Autodesk Inventor part; units mm, degrees
ref_plane "YZ Plane" through (0, 0, 0) normal (1, 0, 0) x (0, 1, 0)
ref_plane "XZ Plane" through (0, 0, 0) normal (0, 1, 0) x (-1, 0, 0)
ref_plane "XY Plane" through (0, 0, 0) normal (0, 0, 1) x (1, 0, 0)
sketch "Sketch1" plane through (0, 0, 0) normal (1, 0, 0) x (0, 1, 0)
  line L0 (0, 0) -> (50.8, 0) construction
  line L1 (50.8, 0) -> (50.8, -25.4) construction
  line L2 (50.8, -25.4) -> (0, -25.4) construction
  line L3 (0, -25.4) -> (0, 0) construction
  line L4 (12.7, -25.4) -> (139.7, -25.4) construction
  line L5 (139.7, -25.4) -> (139.7, -111.252) construction
  line L6 (139.7, -111.252) -> (12.7, -111.252) construction
  line L7 (12.7, -111.252) -> (12.7, -25.4) construction
  line L8 (80.9625, -111.252) -> (665.1625, -111.252) construction
  line L9 (665.1625, -111.252) -> (665.1625, -320.802) construction
  line L10 (665.1625, -320.802) -> (80.9625, -320.802) construction
  line L11 (80.9625, -320.802) -> (80.9625, -111.252) construction
  point P0 (0, -12.7)
  dimension "d0" = 50.8
  dimension "d1" = 25.4
  dimension "d2" = 12.7
  dimension "d3" = 85.852
  dimension "d4" = 127
  dimension "d5" = 80.9625
  dimension "d6" = 209.55
  dimension "d7" = 584.2
sketch "Sketch2" plane through (0, 0, 0) normal (1, 0, 0) x (0, 1, 0)
  line L0 (139.7, -25.4) -> (139.7, -111.252) construction
  line L1 (80.9625, -320.802) -> (80.9625, -111.252) construction
  line L2 (139.7, -111.252) -> (12.7, -111.252) construction
  line L3 (50.8, 0) -> (50.8, -25.4) construction
  line L4 (12.7, -25.4) -> (139.7, -25.4) construction
  line L5 (12.7, -111.252) -> (12.7, -25.4) construction
  line L6 (50.8, -25.4) -> (0, -25.4) construction
  line L7 (0, -25.4) -> (0, 0) construction
  line L8 (0, 0) -> (50.8, 0) construction
  line L9 (665.1625, -320.802) -> (80.9625, -320.802) construction
  line L10 (80.9625, -111.252) -> (665.1625, -111.252) construction
  line L11 (665.1625, -111.252) -> (665.1625, -320.802) construction
  line L12 (50.8, -25.4) -> (190.5, -25.4) construction
  line L13 (190.5, -25.4) -> (190.5, 0) construction
  line L14 (190.5, 0) -> (50.8, 0) construction
  line L15 (50.8, 0) -> (50.8, -25.4) construction
  line L16 (165.1, -12.7) -> (165.1, -216.027) construction
  line L17 (165.1, -216.027) -> (80.9625, -216.027) construction
  line L18 (80.9625, -225.552) -> (174.625, -225.552)
  line L19 (174.625, -225.552) -> (174.625, -12.7)
  line L20 (80.9625, -206.502) -> (155.575, -206.502)
  line L21 (155.575, -206.502) -> (155.575, -12.7)
  line L22 (80.9625, -206.502) -> (80.9625, -225.552)
  arc A0 (174.625, -12.7) -> (155.575, -12.7) centre (165.1, -12.7) ccw
  point P0 (0, -12.7)
  point P1 (190.5, -12.7)
  dimension "d8" = 50.8
  dimension "d9" = 25.4
  dimension "d10" = 9.525
  dimension "d11" = 9.525
  dimension "d12" = 139.7
extrude "Extrusion1" add sketch "Sketch2" along normal blind 6.35
fillet "Fillet1" radius 12.7 2 edges at (3.175, 155.575, -206.502) (3.175, 174.625, -225.552)
fillet "Fillet2" radius 6.604 2 edges at (3.175, 80.9625, -225.552) (3.175, 80.9625, -206.502)
hole "Hole1" at (0, 139.7, -111.252) at (0, 139.7, -25.4) at (0, 80.9625, -111.252) at (0, 80.9625, -320.802) at (0, 50.8, -25.4) at (0, 12.7, -111.252) at (0, 50.8, 0) at (0, 0, -25.4) at (0, 0, -12.7) at (0, 165.1, -12.7) direction (1, 0, 0) diameter 6.7564 end through all
properties part number "CHD-002" material "Aluminum 6061"
For this review, take the finished solid that the model builds, in its own axes (mm). A direction names the side the tool comes from. Round coordinates to 2 decimals unless told otherwise and drop trailing zeros. Order: outer loops, then holes, each group sorted by start corner. A loop starts at its lowest first (then second) coordinate and runs counter-clockwise, first axis right, second up.
Q1. We need section D-D, the plane y = 109.5. Give the boundary of the cut face in (x, z), plus the area to 3 significant figures.
Findings below:
outline: (0, -225.55) - (6.35, -225.55) - (6.35, -206.5) - (0, -206.5) - close
area: 121 mm2
Q2. We need section A-A, the plane y = 165.1. Give the boundary of the cut face in (x, z) (3 decimals), plus the area to 3 significant figures.
Findings below:
outline: (0, -225.149) - (6.35, -225.149) - (6.35, -16.078) - (0, -16.078) - close; (0, -9.322) - (6.35, -9.322) - (6.35, -3.175) - (0, -3.175) - close
area: 1,370 mm2
Q3. Machinability: for faces 4 (the flat face through (6.35, 159, -147)), 5 (the flat face through (3, 155.575, -105)), which of the approach directions +Z, -Z, +X, -X, +Y, -Y give a long, thin tool a straight path to every point of the face, cutting with its end or side? Answer none if there is none.
Findings below:
face 4: +Z, -Z, +X, +Y, -Y
face 5: +Z, +X, -X, -Y
Q4. We need section C-C, the plane z = -161. Give the boundary of the cut face in (x, y) (3 decimals).
Findings below:
outline: (0, 155.575) - (6.35, 155.575) - (6.35, 174.625) - (0, 174.625) - close
Q5. Mouldability with a two-part tool opening along Y and no side actions: class faces 1 (the flat face through (3, 174.625, -114)), 2 (the cylindrical face through (3.22, 168.4, -13.43)), 3 (the cylindrical face through (3.131, 164.891, -3.177)) as pulls with the +Y half, pulls with the -Y half, needs draft (parallel to the pull), parting line crosses it, or undercut.
Findings below:
face 1: pulls with the +Y half
face 2: undercut
face 3: parting line crosses it
Q6. Insertion check: P1, Ø3, axis at x = 2.5, z = -88, coming from the -Y side (3 decimals). The pin has a flat end and moves straight along its axis. Give the tip position at first contact, or say it passes through.
Findings below:
P1: stops at y = 155.575
Q7. Wall thickness on line 1 (Y direction, x = 4.75, z = -12.7) (3 decimals); line 2 (Y direction, x = 3, z = -137.5) (3 decimals); line 3 (Z direction, x = 5.75, y = 115.5): over which ranges is each line inside the solid? List them lowest first.
Findings below:
line 1: y = 155.575 to 161.722, 168.478 to 174.625
line 2: y = 155.575 to 174.625
line 3: z = -225.55 to -206.5
